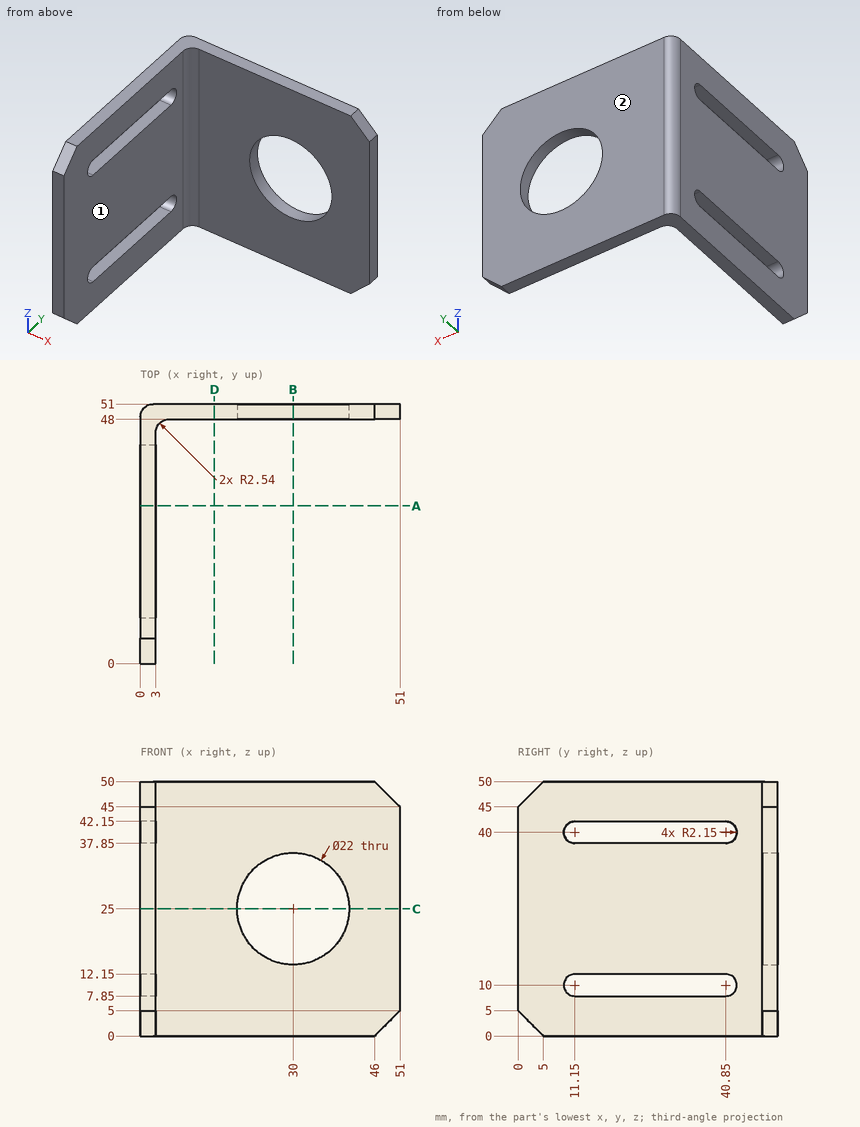
Study the drawing (mm; zero at the part's minimum x, y, z) and answer. A direction names the side the tool comes from. Coordinates: 2 decimals unless noted, no trailing zeros. Loops run counter-clockwise (first coordinate to the right, second up) from the corner with the lowest first, then second, coordinate; pieces in that order, holes last. Notation, with made-up numbers: M 50,59.25 L 107,59.25 A17 cw 107,86.25 Z; hole C -29.75,87.25 d10. An arc over 180 degrees is marked long. Answer in a Markdown table with one row per item. Add a question column.
1. Find section D-D, the plane x = 14.5. Write down the section's boundary in (y, z), then the cut area to 3 significant figures.
2. Find section A-A, the plane y = 31. Write down the section's boundary in (x, z), then the cut area to 3 significant figures.
3. Find section B-B, the plane x = 30. Write down the section's boundary in (y, z), then the cut area to 3 significant figures.
4. A flat-ended cylindrical pin translates along its axis: P1, Ø1, axis at x = 22.5, z = 16, coming from the -Y side. Find the tip coordinate at first contact, or state that the pin passes through.
5. Consider L1, parallel to Z at x = 30, y = 50; L2, parallel to X at y = 44, z = 16; L3, parallel to Y at x = 6, z = 16. Determine where each line is inside the solid, lowest interval first.
6. A tool of negligible diameter and unlimited length cuts with its end or side. For the marked faces 1 and 2, from which of +Z, -Z, +X, -X, +Y, -Y can it reach the whole face along a straight path? Write none if from no direction.
7. Find section C-C, the plane z = 25. Write down the section's boundary in (x, y), then the cut area to 3 significant figures.
Reported:
| question | item | result |
|---|---|---|
| 1 | outline | M 48,0 L 51,0 L 51,50 L 48,50 Z |
| 1 | area | 150 mm^2 |
| 2 | outline | M 0,0 L 3,0 L 3,7.85 L 0,7.85 Z; M 0,12.15 L 3,12.15 L 3,37.85 L 0,37.85 Z; M 0,42.15 L 3,42.15 L 3,50 L 0,50 Z |
| 2 | area | 124 mm^2 |
| 3 | outline | M 48,0 L 51,0 L 51,14 L 48,14 Z; M 48,36 L 51,36 L 51,50 L 48,50 Z |
| 3 | area | 84.0 mm^2 |
| 4 | P1 | stops at y = 48 |
| 5 | L1 | z = 0 to 14, 36 to 50 |
| 5 | L2 | x = 0 to 3 |
| 5 | L3 | y = 48 to 51 |
| 6 | face 1 | +Z, -Z, +X, -Y |
| 6 | face 2 | +Z, -Z, +X, -X, +Y |
| 7 | outline | M 0,0 L 3,0 L 3,45.46 A2.54 cw 5.54,48 L 19,48 L 19,51 L 2.54,51 A2.54 ccw 0,48.46 Z; M 41,48 L 51,48 L 51,51 L 41,51 Z |
| 7 | area | 231 mm^2 |
